For this review, take the finished solid that the model builds, in its own axes (mm). A direction names the side the tool comes from. Coordinates: 2 decimals unless noted, no trailing zeros. Write each loop counter-clockwise with the first axis right and the second up, starting at its lowest first coordinate (ties: lowest second). Pieces come first, ordered by that corner, then holes.
1) Insertion check: P1, Ø6, axis at x = 8, y = 21.5, coming from the +Z side; P2, Ø2, axis at x = 4, z = -5, coming from the +Y side; P3, Ø6, axis at x = 22, z = -16, coming from the +Y side. Each pin has a flat end and moves straight along its axis. Give the tip position at first contact, or say it passes through.
2) To check wall thickness, follow line 1 along Z through (x, y) = (13.5, 13.5); line 2 along Y through (x, z) = (15.5, -2). State the ranges of each line that lie inside material, in increasing order.
3) We need section A-A on y = 15.75. Write out the cut boundary in (x, z).
4) We need section C-C on x = 15. Write out the cut boundary in (y, z), then the cut area to 3 significant figures.
5) We need section D-D on x = 23. Write out the cut boundary in (y, z).
6) Mouldability with a two-part tool opening along X and no side actions: class faces 4 (the face through (26, 14, -10)), 5 (the face through (25, 15, -20)), 6 (the face through (0, 15, -18)) as pulls with the +X half, pulls with the -X half, needs draft (parallel to the pull), parting line crosses it, or undercut.
7) We need section B-B on z = -24. Write out the cut boundary in (x, y), then the cut area to 3 significant figures.
8) For faces 1 (the face through (15, 15, -20)), 2 (the face through (6, 18, -10)), 3 (the face through (10, 25, -20)), list the 3-axis set-ups (+Z, -Z, +X, -X, +Y, -Y) from which the entire face can be reached by the end or side of a thin tool; tool diameter is ignored.
from build123d import *

# Parameters (mm, degrees)
SKETCH_1_W           = 30
SKETCH_1_H           = 30
EXTRUDE_1_DEPTH      = 30
SKETCH_28_W          = 20
SKETCH_28_H          = 10
CUT_EXTRUDE_18_DEPTH = 52.961524227
SKETCH_29_W          = 10
SKETCH_29_H          = 10
CUT_EXTRUDE_19_DEPTH = 52.961524227


with BuildPart() as part:
    # 草圖1 → 填料-伸1 (new body)
    with BuildSketch(Plane.XY):
        with Locations((15, 15)):
            Rectangle(SKETCH_1_W, SKETCH_1_H)
    extrude(amount=-EXTRUDE_1_DEPTH)

    # 草圖28 → 除料-伸長18 (cut, through all)
    with BuildSketch(Plane.XY):
        with Locations((20, 25)):
            Rectangle(SKETCH_28_W, SKETCH_28_H)
        Polygon((10, 20), (30, 20), (20, 10), align=None)
    extrude(amount=-CUT_EXTRUDE_18_DEPTH, mode=Mode.SUBTRACT)

    # 草圖29 → 除料-伸長19 (cut, through all)
    with BuildSketch(Plane(origin=(30, 0, 0), x_dir=(0, 0, -1), z_dir=(1, 0, 0))):
        with Locations((5, 25)):
            Rectangle(SKETCH_29_W, SKETCH_29_H)
        with Locations((5, 15)):
            Rectangle(SKETCH_29_W, SKETCH_29_H)
    extrude(amount=-CUT_EXTRUDE_19_DEPTH, mode=Mode.SUBTRACT)


solid = part.part
Result:
1. P1: stops at z = -10
1. P2: stops at y = 10
1. P3: stops at y = 15
2. line 1: z = -30 to -10
2. line 2: y = 0 to 10
3. outline: (0, -30) - (14.25, -30) - (14.25, -10) - (0, -10) - close; (25.75, -30) - (30, -30) - (30, -10) - (25.75, -10) - close
4. outline: (0, -30) - (15, -30) - (15, -10) - (10, -10) - (10, 0) - (0, 0) - close
4. area: 400 mm2
5. outline: (0, -30) - (13, -30) - (13, -10) - (10, -10) - (10, 0) - (0, 0) - close
6. face 4: needs draft
6. face 5: undercut
6. face 6: pulls with the -X half
7. outline: (0, 0) - (30, 0) - (30, 20) - (20, 10) - (10, 20) - (10, 30) - (0, 30) - close
7. area: 600 mm2
8. face 1: +Z, -Z, +Y
8. face 2: +Z, +X, -X, +Y
8. face 3: +Z, -Z, +X, +Y
